Design review of the part built by this model. Coordinates are the model's own, in mm. Round coordinates to 2 decimals unless told otherwise and drop trailing zeros. Loops run counter-clockwise (first coordinate to the right, second up) from the corner with the lowest first, then second, coordinate; pieces in that order, holes last. Notation, with made-up numbers: M 57.25,36.25 L 98.25,36.25 A35 ccw 98.25,72.25 Z; hole C 23.25,-5 d4. An arc over 180 degrees is marked long. Answer as CSV lines item,"result". Start each with the question number.
from build123d import *

# Parameters (mm, degrees)
EXTRUDE1_START = -5
SKETCH1_R      = 15
SKETCH1_R_2    = 7.95
EXTRUDE1_DEPTH = 10
CHAMFER1_SIZE  = 0.3


with BuildPart() as part:
    # Sketch1 → Extrude1 (new body)
    with BuildSketch(Plane.XY.offset(EXTRUDE1_START)):
        Circle(SKETCH1_R)
        Circle(SKETCH1_R_2, mode=Mode.SUBTRACT)
    extrude(amount=EXTRUDE1_DEPTH)

    # Chamfer1
    chamfer1_edges = [part.edges().sort_by_distance(p)[0] for p in [
        (-15, 0, -5),
        (-15, 0, 5),
    ]]
    chamfer(chamfer1_edges, length=CHAMFER1_SIZE)

    # Sketch2 → Revolve1 (revolve)
    with BuildSketch(Plane(origin=(0, 0, 0), x_dir=(0, 0, -1), z_dir=(1, 0, 0))):
        with BuildLine():
            Line((7, 3), (-7, 3))
            Line((-7, 3), (-7, 10.596697599))
            ThreePointArc((-7, 10.596697599), (0, 12.7), (7, 10.596697599))
            Line((7, 10.596697599), (7, 3))
        make_face()
    revolve(axis=Axis((0, 0, -11.466432169), (0, 0, 1)))

    # Sketch2_2 → Cut-Revolve1 (revolve, cut)
    with BuildSketch(Plane(origin=(0, 0, 0), x_dir=(0, 0, -1), z_dir=(1, 0, 0))):
        with BuildLine():
            Line((7, 3), (-7, 3))
            Line((-7, 3), (-7, 10.596697599))
            ThreePointArc((-7, 10.596697599), (0, 12.7), (7, 10.596697599))
            Line((7, 10.596697599), (7, 3))
        make_face()
    revolve(axis=Axis((0, 0, -11.466432169), (0, 0, 1)), mode=Mode.SUBTRACT)


solid = part.part
Item 1: To check wall thickness, follow line 1 (Y direction, x = -11, z = 0.25); line 2 (Y direction, x = 2, z = 2.25); line 3 (X direction, y = -6, z = 2.5). State the ranges of each line that lie inside material, in increasing order.
Item 2: Insertion check: pin 1 Ø3 at (x, z) = (8.5, -2) entering from -Y; pin 2 Ø1 at (y, z) = (-7.5, -2) entering from +X; pin 3 Ø3 at (x, z) = (-2, 1) entering from +Y. Each pin has a flat end and moves straight along its axis. Give the tip position at first contact, or say it passes through.
Item 3: Consider section A-A, the plane x = 0. Write out the cut boundary in (y, z).
Item 4: Consider section C-C, the plane z = -1.5. Write out the cut boundary in (x, y), then the cut area to 3 significant figures.
Found:
1,line 1,"y = -10.2 to -6.34, 6.34 to 10.2"
1,line 2,"y = -14.87 to -12.34, 12.34 to 14.87"
1,line 3,"x = -13.75 to -10.91, 10.91 to 13.75"
2,pin 1,"stops at y = -13.27"
2,pin 2,"stops at x = 13.27"
2,pin 3,"stops at y = 14.99"
3,outline,"M -15,-4.7 L -14.7,-5 L -11.67,-5 A12.7 cw -11.67,5 L -14.7,5 L -15,4.7 Z; M 11.67,-5 L 14.7,-5 L 15,-4.7 L 15,4.7 L 14.7,5 L 11.67,5 A12.7 cw Z"
4,outline,"C 0,0 d30; hole C 0,0 d25.22"
4,area,"207 mm^2"
